Could you check a few things on this model? Use its own coordinates, in mm. Face numbers are marked on the shaded views. A direction names the side the tool comes from. Give positions to 0.01 mm unless a question says otherwise; leave off trailing zeros. Write each loop counter-clockwise with the first axis right and the second up, starting at its lowest first coordinate (ties: lowest second). Pieces come first, ordered by that corner, then holes. Notation, with made-up numbers: M -17,73.25 L -3,73.25 A28 ccw -3,107.25 Z; hole C -20.75,-26.75 d9. An arc over 180 degrees is marked long. Use one line per item in the form item = value.
from build123d import *

# Parameters (mm, degrees)
BOSS_EXTRUDE1_DEPTH = 2.794
SKETCH2_R           = 3.81
BOSS_EXTRUDE2_DEPTH = 0.8128
SKETCH3_R           = 1.3843
BOSS_EXTRUDE3_DEPTH = 25.4


with BuildPart() as part:
    # Sketch1 → Boss-Extrude1 (new body)
    with BuildSketch(Plane.XY):
        Polygon((2.756963005, 0), (1.378481503, 2.3876), (-1.378481503, 2.3876), (-2.756963005, 0), (-1.378481503, -2.3876), (1.378481503, -2.3876), align=None)
    extrude(amount=BOSS_EXTRUDE1_DEPTH)

    # Sketch2 → Boss-Extrude2 (add)
    with BuildSketch(Plane.XY.offset(2.794)):
        Circle(SKETCH2_R)
    extrude(amount=BOSS_EXTRUDE2_DEPTH)

    # Sketch3 → Boss-Extrude3 (add)
    with BuildSketch(Plane.XY.offset(3.6068)):
        Circle(SKETCH3_R)
    extrude(amount=BOSS_EXTRUDE3_DEPTH)


solid = part.part
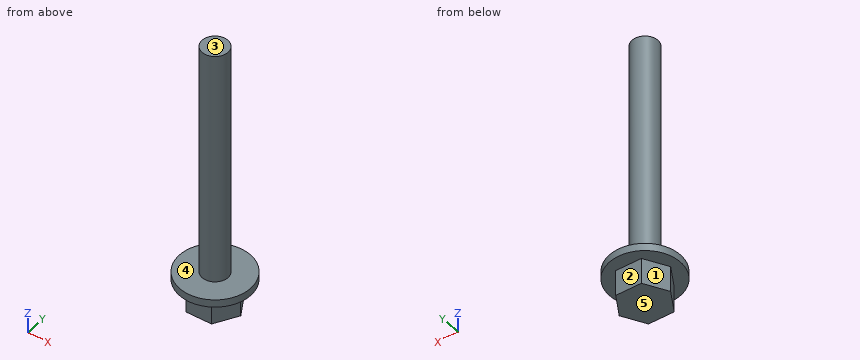
1) For pin 1 Ø4 at (x, y) = (0, 1.5) entering from +Z; pin 2 Ø4 at (y, z) = (0.5, 12.5) entering from +X; pin 3 Ø1.4 at (x, z) = (-0.5, 1) entering from +Y; pin 4 Ø4 at (x, z) = (-0.5, 22) entering from +Y, each with a flat end and sliding along its axis, tell me the tip position at first contact or that it passes through.
Checked values:
pin_1 = 29.01
pin_2 = 1.38
pin_3 = 2.39
pin_4 = 1.38
2) I want a section at A-A, the plane x = 0. Please give me the cut outline in (y, z).
Checked values:
outline = M -3.81,2.79 L -2.39,2.79 L -2.39,0 L 2.39,0 L 2.39,2.79 L 3.81,2.79 L 3.81,3.61 L 1.38,3.61 L 1.38,29.01 L -1.38,29.01 L -1.38,3.61 L -3.81,3.61 Z
3) I want a section at C-C, the plane z = 23.25. Please give me the cut outline in (x, y), plus the area to 3 significant figures.
Checked values:
outline = C 0,0 d2.77
area = 6.02 mm2
4) For the marked faces 1, 2, 3, 4 and 5, which set-ups out of +Z, -Z, +X, -X, +Y, -Y let a thin tool reach every point of the face, with its end or its side?
Checked values:
face_1 = -Z, -X, +Y
face_2 = -Z, +X, -X, +Y
face_3 = +Z, +X, -X, +Y, -Y
face_4 = +Z
face_5 = -Z, +X, -X, +Y, -Y
5) If I drill on L1, parallel to Z at x = 2.25, y = 0.5; L2, parallel to Z at x = 0, y = 2.75; L3, parallel to Y at x = 0, z = 6.75, over which ranges is the centre line in solid material (lowest first)?
Checked values:
L1 = 0 to 3.61
L2 = 2.79 to 3.61
L3 = -1.38 to 1.38
6) I want a section at D-D, the plane x = 2.25. Please give me the cut outline in (y, z).
Checked values:
outline = M -3.07,2.79 L -0.88,2.79 L -0.88,0 L 0.88,0 L 0.88,2.79 L 3.07,2.79 L 3.07,3.61 L -3.07,3.61 Z
7) I want a section at B-B, the plane y = 0.5. Please give me the cut outline in (x, z).
Checked values:
outline = M -3.78,2.79 L -2.47,2.79 L -2.47,0 L 2.47,0 L 2.47,2.79 L 3.78,2.79 L 3.78,3.61 L 1.29,3.61 L 1.29,29.01 L -1.29,29.01 L -1.29,3.61 L -3.78,3.61 Z
